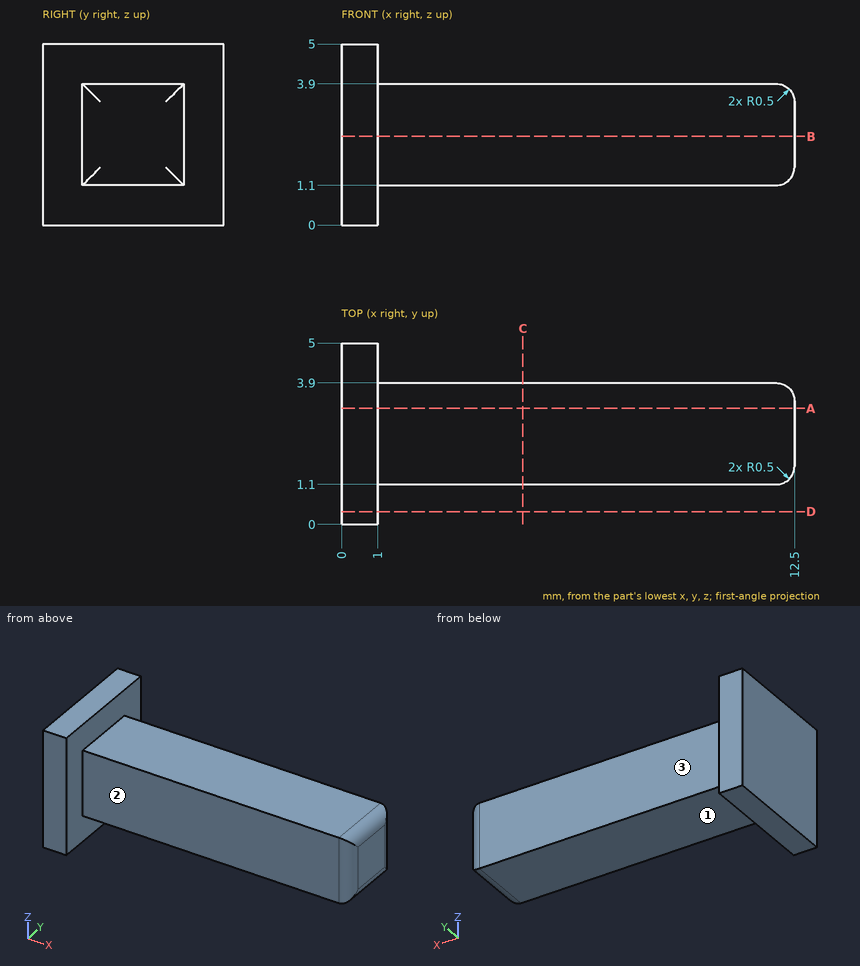
Part print with two shaded views. Sizes in mm from the minimum x, y, z corner. A direction names the side the tool comes from. Give positions to 0.01 mm unless a question says otherwise; leave off trailing zeros. Write each loop counter-clockwise with the first axis right and the second up, starting at its lowest first coordinate (ties: lowest second). Pieces come first, ordered by that corner, then holes.
1) Cut at D-D on y = 0.35. Write the cut outline in (x, z).
Resolved:
outline: (0, 0) - (1, 0) - (1, 5) - (0, 5) - close
2) Which spindle directions (+Z, -Z, +X, -X, +Y, -Y) get a long thin tool onto all of the face, cutting with end or side? Do the marked faces 1, 2 and 3. Say none if no direction does.
Resolved:
face 1: -Z, +X, +Y, -Y
face 2: +Z, -Z, +X, -Y
face 3: +Z, -Z, +X, +Y
3) Probe L1, parallel to Z at x = 11, y = 3.5; L2, parallel to X at y = 4.55, z = 3.6. List the from-to ranges inside material, lowest first.
Resolved:
L1: z = 1.1 to 3.9
L2: x = 0 to 1
4) Cut at A-A on y = 3.2. Write the cut outline in (x, z).
Resolved:
outline: (0, 0) - (1, 0) - (1, 1.1) - (12, 1.1) arc R0.5 ccw to (12.5, 1.6) - (12.5, 3.4) arc R0.5 ccw to (12, 3.9) - (1, 3.9) - (1, 5) - (0, 5) - close
5) Pin check, flat tips, straight feed: pin 1 (1.4 mm diameter, centred on x = 5.5, z = 2, fed in from +Y); pin 2 (1 mm diameter, centred on x = 5.5, z = 4, fed in from -Y); pin 3 (1.5 mm diameter, centred on x = 9.5, y = 0.5, fed in from -Z). Stop position of each tip, or through.
Resolved:
pin 1: stops at y = 3.9
pin 2: stops at y = 1.1
pin 3: stops at z = 1.1
6) Cut at C-C on x = 5. Write the cut outline in (y, z).
Resolved:
outline: (1.1, 1.1) - (3.9, 1.1) - (3.9, 3.9) - (1.1, 3.9) - close
